Geometry check sheet. Reference: drawing and pictorial views, mm from the part's lowest x, y, z. Round coordinates to 2 decimals unless told otherwise and drop trailing zeros. Loops run counter-clockwise (first coordinate to the right, second up) from the corner with the lowest first, then second, coordinate; pieces in that order, holes last. Notation, with made-up numbers: (57, 15.5) - (82, 15.5) arc R24 cw to (82, 42.5) - close; hole circle Ø6 at (-24.5, -14.5). An arc over 180 degrees is marked (long way). Put each result on its own line as item: value. Start each with the question number.
Item 1: Section check B-B, the plane z = 0.8. Give the number of separate pieces and of enclosed holes in the cut face, and give its area (3 significant figures).
Item 2: Section check A-A, the plane y = 23.5. Record the cut outline in (x, z) (1 decimal).
Item 3: Section check C-C, the plane x = 30.5. Record the cut outline in (y, z).
Item 4: Material ranges on line 1 along Y through (x, z) = (28.5, 1.05) (1 decimal); line 2 along Y through (x, z) = (23.5, 1.45); line 3 along Y through (x, z) = (35.5, 0.65), recorded low to high.
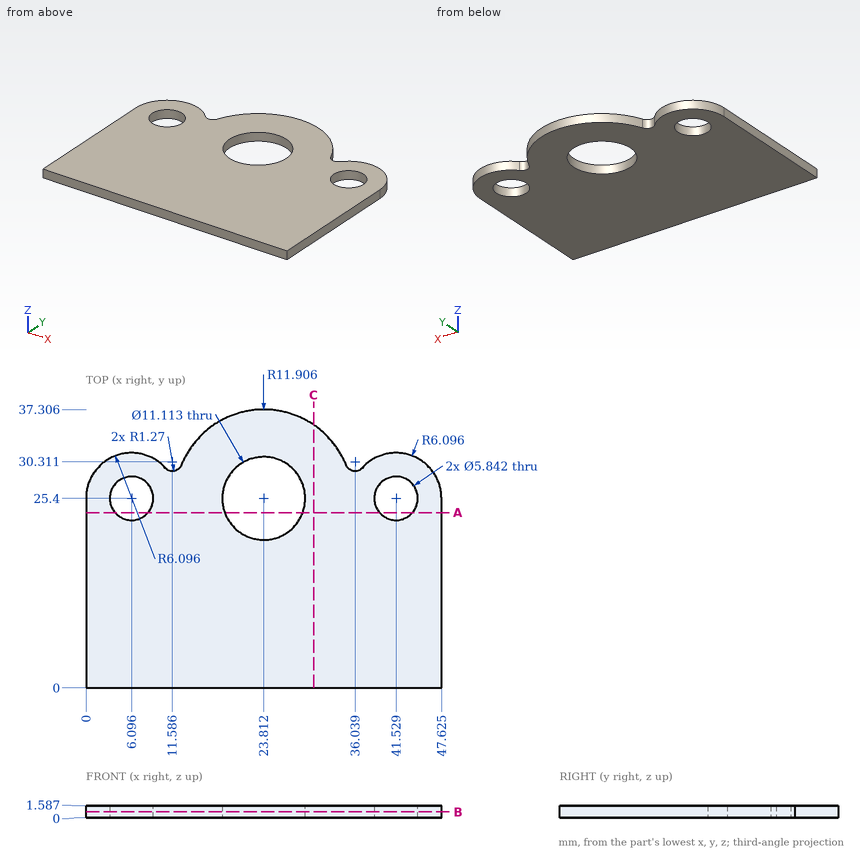
Check result:
1. separate pieces: 1
1. enclosed holes: 3
1. area: 1,400 mm²
2. outline: (0, 0) - (3.9, 0) - (3.9, 1.6) - (0, 1.6) - close; (8.3, 0) - (18.6, 0) - (18.6, 1.6) - (8.3, 1.6) - close; (29, 0) - (39.3, 0) - (39.3, 1.6) - (29, 1.6) - close; (43.7, 0) - (47.6, 0) - (47.6, 1.6) - (43.7, 1.6) - close
3. outline: (0, 0) - (35.25, 0) - (35.25, 1.59) - (0, 1.59) - close
4. line 1: 0 to 22.4, 28.4 to 36.3
4. line 2: 0 to 19.85, 30.95 to 37.3
4. line 3: 0 to 29.16
